from build123d import *

# Parameters (mm, degrees)
BOSS_EXTRUDE1_DEPTH = 5
CUT_EXTRUDE2_DEPTH  = 16
SKETCH3_R           = 0.75
CUT_EXTRUDE3_DEPTH  = 8


with BuildPart() as part:
    # Sketch1 → Boss-Extrude1 (new body)
    with BuildSketch(Plane.XY):
        with BuildLine():
            Line((-11.358992197, -0.975163345), (-11.358992197, 0.975163345))
            ThreePointArc((-11.358992197, 0.975163345), (-10.949461796, 2.187766517), (-9.888585744, 2.903771827))
            Line((-9.888585744, 2.903771827), (4.032865761, 6.726585506))
            ThreePointArc((4.032865761, 6.726585506), (5.035336984, 6.894716557), (6.051095895, 6.856631946))
            Line((6.051095895, 6.856631946), (19.293138558, 5))
            ThreePointArc((19.293138558, 5), (23.641007803, 0), (19.293138558, -5))
            Line((19.293138558, -5), (6.051095895, -6.856631946))
            ThreePointArc((6.051095895, -6.856631946), (5.035336984, -6.894716557), (4.032865761, -6.726585506))
            Line((4.032865761, -6.726585506), (-9.888585744, -2.903771827))
            ThreePointArc((-9.888585744, -2.903771827), (-10.949461796, -2.187766517), (-11.358992197, -0.975163345))
        make_face()
    extrude(amount=BOSS_EXTRUDE1_DEPTH)

    # Sketch2 → Cut-Extrude2 (cut)
    with BuildSketch(Plane.ZY.offset(11.358992197)):
        with BuildLine():
            Line((1, -0.745034354), (1, 0.754965646))
            Line((1, 0.754965646), (3, 0.754965646))
            ThreePointArc((3, 0.754965646), (3.75, 0.004965646), (3, -0.745034354))
            Line((3, -0.745034354), (1, -0.745034354))
        make_face()
    extrude(amount=-CUT_EXTRUDE2_DEPTH, mode=Mode.SUBTRACT)

    # Sketch3 → Cut-Extrude3 (cut)
    with BuildSketch(Plane.XY.offset(5)):
        with Locations((18.592101719, 0)):
            Circle(SKETCH3_R)
        with Locations((10.592101719, 0)):
            Circle(SKETCH3_R)
    extrude(amount=-CUT_EXTRUDE3_DEPTH, mode=Mode.SUBTRACT)


solid = part.part
Geometry: final body of the model. Coordinates: model frame, mm. A direction names the side the tool comes from. Give positions to 0.01 mm unless a question says otherwise; leave off trailing zeros. Write each loop counter-clockwise with the first axis right and the second up, starting at its lowest first coordinate (ties: lowest second). Pieces come first, ordered by that corner, then holes. Notation, with made-up numbers: (15, 69) -> (59, 69) arc R8 cw to (59, 78) -> close; hole circle Ø2 at (-7, 63). An arc over 180 degrees is marked (long way). Answer as a JSON object with one key per item and string values.
1. Cut plane B-B on y = 0. Output: boundary loops of the cut face in (x, z).
Ans:
{"outline": "(-11.36, 0) -> (9.84, 0) -> (9.84, 5) -> (-11.36, 5) -> (-11.36, 3.75) -> (4.64, 3.75) -> (4.64, 1) -> (-11.36, 1) -> close; (11.34, 0) -> (17.84, 0) -> (17.84, 5) -> (11.34, 5) -> close; (19.34, 0) -> (23.64, 0) -> (23.64, 5) -> (19.34, 5) -> close"}
2. Ray query, probe 1 along Y at (x, z) = (10.5, 3.1); probe 2 along Y at (x, z) = (4.5, 2.3); probe 3 along Y at (x, z) = (17, 2.2). Return the intervals inside material, ascending. Write a range as from..to.
Ans:
{"probe 1": "y = -6.23..-0.74, 0.74..6.23", "probe 2": "y = -6.83..-0.75, 0.75..6.83", "probe 3": "y = -5.32..5.32"}
3. Contact query for flat-ended pins moving along their axis: pin 1 (0.6 mm diameter, centred on x = -3.5, z = 2, fed in from -Y); pin 2 (1.5 mm diameter, centred on y = 4, z = 1.5, fed in from +X); pin 3 (0.6 mm diameter, centred on x = -2, z = 1.5, fed in from +Y); pin 4 (1.4 mm diameter, centred on x = 10.59, y = 0, fed in from +Z). Output: stop coordinate, or through.
Ans:
{"pin 1": "stops at y = -4.74", "pin 2": "stops at x = 22.46", "pin 3": "stops at y = 5.15", "pin 4": "passes through"}
4. Access query for faces 4 (the flat face through (4.641, 0, 2)), 5 (the flat face through (6, 0, 5)). Directions: +Z, -Z, +X, -X, +Y, -Y. A direction counts if a zero-diameter tool reaches every point of the face in a straight line with its end or side. Return the directions, or none.
Ans:
{"face 4": "-X", "face 5": "+Z, +X, -X, +Y, -Y"}
5. Cut plane C-C on x = -6.5. Output: boundary loops of the cut face in (y, z).
Ans:
{"outline": "(-3.83, 0) -> (3.83, 0) -> (3.83, 5) -> (-3.83, 5) -> close; hole (-0.75, 1) -> (0.75, 1) -> (0.75, 3) arc R0.75 ccw to (-0.75, 3) -> close"}
6. Mould query, pull axis X, two halves, no side actions, for faces 1 (the cylindrical face through (19.307, 0.225, 2.535)), 2 (the cylindrical face through (5.05, -6.896, 2.465)), 3 (the flat face through (-3.025, 4.788, 2.465)). Classes: pulls with the +X half, pulls with the -X half, needs draft (parallel to the pull), parting line crosses it, or undercut.
Ans:
{"face 1": "undercut", "face 2": "parting line crosses it", "face 3": "pulls with the -X half"}
7. Cut plane A-A on z = 0.6. Output: boundary loops of the cut face in (x, y), and give its area (3 significant figures).
Ans:
{"outline": "(-11.36, -0.98) arc R2 ccw to (-9.89, -2.9) -> (4.03, -6.73) arc R5 ccw to (6.05, -6.86) -> (19.29, -5) arc R5.05 ccw to (19.29, 5) -> (6.05, 6.86) arc R5 ccw to (4.03, 6.73) -> (-9.89, 2.9) arc R2 ccw to (-11.36, 0.98) -> close; hole circle Ø1.5 at (10.59, 0); hole circle Ø1.5 at (18.59, 0)", "area": "355 mm^2"}
8. Cut plane D-D on z = 2.3. Output: boundary loops of the cut face in (x, y), and give its area (3 significant figures).
Ans:
{"outline": "(-11.36, -0.98) arc R2 ccw to (-9.89, -2.9) -> (4.03, -6.73) arc R5 ccw to (6.05, -6.86) -> (19.29, -5) arc R5.05 ccw to (19.29, 5) -> (6.05, 6.86) arc R5 ccw to (4.03, 6.73) -> (-9.89, 2.9) arc R2 ccw to (-11.36, 0.98) -> (-11.36, 0.75) -> (4.64, 0.75) -> (4.64, -0.75) -> (-11.36, -0.75) -> close; hole circle Ø1.5 at (10.59, 0); hole circle Ø1.5 at (18.59, 0)", "area": "331 mm^2"}
